from build123d import *

# Parameters (mm, degrees)
SKETCH1_W           = 45
SKETCH1_H           = 6
BOSS_EXTRUDE1_DEPTH = 32
SKETCH2_W           = 23.1
SKETCH2_H           = 17.6
CUT_EXTRUDE1_DEPTH  = 56.542776308
SKETCH3_W           = 45
SKETCH3_H           = 20
BOSS_EXTRUDE2_DEPTH = 6
SKETCH4_W           = 20
SKETCH4_H           = 6
BOSS_EXTRUDE3_DEPTH = 30
SKETCH5_R           = 1.4
CUT_EXTRUDE2_DEPTH  = 87.423376467
BOSS_EXTRUDE4_DEPTH = 7
SKETCH7_W           = 32
SKETCH7_H           = 2.5
CUT_EXTRUDE3_DEPTH  = 17.6
SKETCH8_R           = 1.35
CUT_EXTRUDE4_DEPTH  = 86.895285086
CHAMFER1_SIZE       = 1
FILLET1_R           = 1


with BuildPart() as part:
    # Sketch1 → Boss-Extrude1 (new body)
    with BuildSketch(Plane(origin=(0, 0, 0), x_dir=(1, 0, 0), z_dir=(0, 1, 0))):
        with Locations((22.5, 3)):
            Rectangle(SKETCH1_W, SKETCH1_H)
    extrude(amount=BOSS_EXTRUDE1_DEPTH)

    # Sketch2 → Cut-Extrude1 (cut, through all)
    with BuildSketch(Plane.XY):
        with Locations((22.5, 23.2)):
            Rectangle(SKETCH2_W, SKETCH2_H)
    extrude(amount=-CUT_EXTRUDE1_DEPTH, mode=Mode.SUBTRACT)

    # Sketch3 → Boss-Extrude2 (add)
    with BuildSketch(Plane.XZ):
        with Locations((22.5, -10)):
            Rectangle(SKETCH3_W, SKETCH3_H)
    extrude(amount=BOSS_EXTRUDE2_DEPTH)

    # Sketch4 → Boss-Extrude3 (add)
    with BuildSketch(Plane(origin=(45, 0, 0), x_dir=(0, 0, -1), z_dir=(1, 0, 0))):
        with Locations((10, -3)):
            Rectangle(SKETCH4_W, SKETCH4_H)
    extrude(amount=BOSS_EXTRUDE3_DEPTH)

    # Sketch5 → Cut-Extrude2 (cut, through all)
    with BuildSketch(Plane.XZ.offset(6)):
        with Locations(Location((37.288839919, -16.75, 0), (0, 0, 270))):
            Circle(SKETCH5_R)
        with Locations(Location((47.288839919, -16.75, 0), (0, 0, 270))):
            Circle(SKETCH5_R)
        with Locations(Location((47.288839919, -6.75, 0), (0, 0, 270))):
            Circle(SKETCH5_R)
        with Locations(Location((59.538839919, -16.75, 0), (0, 0, 270))):
            Circle(SKETCH5_R)
        with Locations(Location((71.788839919, -16.75, 0), (0, 0, 270))):
            Circle(SKETCH5_R)
        with Locations(Location((71.788839919, -6.75, 0), (0, 0, 270))):
            Circle(SKETCH5_R)
        with Locations(Location((59.538839919, -6.75, 0), (0, 0, 270))):
            Circle(SKETCH5_R)
    extrude(amount=-CUT_EXTRUDE2_DEPTH, mode=Mode.SUBTRACT)

    # Sketch6 → Boss-Extrude4 (add)
    with BuildSketch(Plane.XY):
        Polygon((0, 32), (0, -6), (45, -6), (45, 0), (45, 32), (34.05, 32), (34.05, 14.4), (10.95, 14.4), (10.95, 32), align=None)
    extrude(amount=BOSS_EXTRUDE4_DEPTH)

    # Sketch7 → Cut-Extrude3 (cut)
    with BuildSketch(Plane(origin=(0, 32, 0), x_dir=(1, 0, 0), z_dir=(0, 1, 0))):
        with Locations((22.5, -1.25)):
            Rectangle(SKETCH7_W, SKETCH7_H)
    extrude(amount=-CUT_EXTRUDE3_DEPTH, mode=Mode.SUBTRACT)

    # Sketch8 → Cut-Extrude4 (cut, through all)
    with BuildSketch(Plane.XY.offset(7)):
        with Locations((8.45, 28)):
            Circle(SKETCH8_R)
        with Locations((36.55, 28)):
            Circle(SKETCH8_R)
    extrude(amount=-CUT_EXTRUDE4_DEPTH, mode=Mode.SUBTRACT)

    # Chamfer1
    chamfer1_edges = [part.edges().sort_by_distance(p)[0] for p in [
        (22.5, -6, 7),
        (0, -6, -6.5),
        (37.5, -6, -20),
        (60, -6, 0),
        (75, -6, -10),
        (45, -6, 3.5),
    ]]
    chamfer(chamfer1_edges, length=CHAMFER1_SIZE)

    # Fillet1
    # the kernel refuses this fillet: 1 mm, written as the material it adds along each edge
    with BuildSketch(Plane(origin=(45, 0, -6), x_dir=(0, 1, 0), z_dir=(0, 0, 1))) as fillet1_piece_1:
        with BuildLine():
            CenterArc((FILLET1_R, -FILLET1_R), FILLET1_R, 90, 90)
            Line((0, -FILLET1_R), (0, 0))
            Line((0, 0), (FILLET1_R, 0))
        make_face()
    extrude(amount=6)
    with BuildSketch(Plane(origin=(45, 0, -6), x_dir=(0, 0, -1), z_dir=(-1, 0, 0))) as fillet1_piece_2:
        with BuildLine():
            CenterArc((FILLET1_R, -FILLET1_R), FILLET1_R, 90, 90)
            Line((0, -FILLET1_R), (0, 0))
            Line((0, 0), (FILLET1_R, 0))
        make_face()
    extrude(amount=45)
    with BuildSketch(Plane(origin=(45, -7.5, 0), x_dir=(1, 0, 0), z_dir=(0, 1, 0))) as fillet1_piece_3_section:
        with BuildLine():
            CenterArc((FILLET1_R, -FILLET1_R), FILLET1_R, 90, 90)
            Line((0, -FILLET1_R), (0, 0))
            Line((0, 0), (FILLET1_R, 0))
        make_face()
    fillet1_piece_3 = extrude(amount=7.5, mode=Mode.PRIVATE)
    fillet1_piece_3 = split(fillet1_piece_3, bisect_by=Plane(origin=(45.042981958, -4.592558865, 0.407441135), z_dir=(0, -0.7071067811865476, 0.7071067811865476)), keep=Keep.TOP, mode=Mode.PRIVATE)
    fillet1_piece_3 = split(fillet1_piece_3, bisect_by=Plane(origin=(45.16446835, -4.83553165, 0.528927527), z_dir=(-0.7071067811865476, 0.7071067811865476, 0)), keep=Keep.TOP, mode=Mode.PRIVATE)
    add(fillet1_piece_3)
    with BuildSketch(Plane(origin=(45, -7.5, 0), x_dir=(1, 0, 0), z_dir=(0, 1, 0))) as fillet1_piece_4_section:
        with BuildLine():
            CenterArc((FILLET1_R, -FILLET1_R), FILLET1_R, 90, 90)
            Line((0, -FILLET1_R), (0, 0))
            Line((0, 0), (FILLET1_R, 0))
        make_face()
    fillet1_piece_4 = extrude(amount=7.5, mode=Mode.PRIVATE)
    fillet1_piece_4 = split(fillet1_piece_4, bisect_by=Plane(origin=(45.528927527, -4.83553165, 0.16446835), z_dir=(0, 0.7071067811865476, -0.7071067811865476)), keep=Keep.TOP, mode=Mode.PRIVATE)
    fillet1_piece_4 = split(fillet1_piece_4, bisect_by=Plane(origin=(45.407441135, -4.592558865, 0.042981958), z_dir=(0.7071067811865476, -0.7071067811865476, 0)), keep=Keep.TOP, mode=Mode.PRIVATE)
    add(fillet1_piece_4)
    with BuildSketch(Plane(origin=(45, -7.5, 0), x_dir=(1, 0, 0), z_dir=(0, 1, 0))) as fillet1_piece_5_section:
        with BuildLine():
            CenterArc((FILLET1_R, -FILLET1_R), FILLET1_R, 90, 90)
            Line((0, -FILLET1_R), (0, 0))
            Line((0, 0), (FILLET1_R, 0))
        make_face()
    fillet1_piece_5 = extrude(amount=7.5, mode=Mode.PRIVATE)
    fillet1_piece_5 = split(fillet1_piece_5, bisect_by=Plane(origin=(45.222376568, -3.546419499, 1.453580501), z_dir=(0, 0.7071067811865476, -0.7071067811865476)), keep=Keep.TOP, mode=Mode.PRIVATE)
    fillet1_piece_5 = split(fillet1_piece_5, bisect_by=Plane(origin=(46.453580501, -3.546419499, 0.222376568), z_dir=(-0.7071067811865476, 0.7071067811865476, 0)), keep=Keep.TOP, mode=Mode.PRIVATE)
    add(fillet1_piece_5)
    with BuildSketch(Plane(origin=(45, 0, -8.5), x_dir=(0, 1, 0), z_dir=(0, 0, 1))) as fillet1_piece_6a_section:
        with BuildLine():
            CenterArc((FILLET1_R, -FILLET1_R), FILLET1_R, 90, 90)
            Line((0, -FILLET1_R), (0, 0))
            Line((0, 0), (FILLET1_R, 0))
        make_face()
    fillet1_piece_6a = extrude(amount=8.5, mode=Mode.PRIVATE)
    fillet1_piece_6a = split(fillet1_piece_6a, bisect_by=Plane(origin=(45.224393795, 0.227043758, -6), z_dir=(0, 0, -1)), keep=Keep.TOP, mode=Mode.PRIVATE)
    fillet1_piece_6a = fillet1_piece_6a - Plane(origin=(47.288839919, 0.227043758, -6.75), x_dir=(0, 0, -1), z_dir=(0, -1, 0)) * Cylinder(1.4, 21, mode=Mode.PRIVATE)
    with BuildSketch(Plane(origin=(47.5, 0, -6), x_dir=(0, 0, -1), z_dir=(-1, 0, 0))) as fillet1_piece_6b_section:
        with BuildLine():
            CenterArc((FILLET1_R, -FILLET1_R), FILLET1_R, 90, 90)
            Line((0, -FILLET1_R), (0, 0))
            Line((0, 0), (FILLET1_R, 0))
        make_face()
    fillet1_piece_6b = extrude(amount=47.5, mode=Mode.PRIVATE)
    fillet1_piece_6b = split(fillet1_piece_6b, bisect_by=Plane(origin=(45, 0.236066937, -6.212082633), z_dir=(1, 0, 0)), keep=Keep.TOP, mode=Mode.PRIVATE)
    fillet1_piece_6b = fillet1_piece_6b - Plane(origin=(47.288839919, 0.236066937, -6.75), x_dir=(0, 0, -1), z_dir=(0, -1, 0)) * Cylinder(1.4, 99, mode=Mode.PRIVATE)
    fillet1_piece_6 = fillet1_piece_6a & fillet1_piece_6b
    add(fillet1_piece_6)
    with BuildSketch(Plane(origin=(45, -7.5, 0), x_dir=(1, 0, 0), z_dir=(0, 1, 0))) as fillet1_piece_7a_section:
        with BuildLine():
            CenterArc((FILLET1_R, -FILLET1_R), FILLET1_R, 90, 90)
            Line((0, -FILLET1_R), (0, 0))
            Line((0, 0), (FILLET1_R, 0))
        make_face()
    fillet1_piece_7a = extrude(amount=10, mode=Mode.PRIVATE)
    fillet1_piece_7a = split(fillet1_piece_7a, bisect_by=Plane(origin=(45.226395114, 0, 0.226395114), z_dir=(0, 1, 0)), keep=Keep.TOP, mode=Mode.PRIVATE)
    with BuildSketch(Plane(origin=(45, 0, -6), x_dir=(0, 1, 0), z_dir=(0, 0, 1))) as fillet1_piece_7b_section:
        with BuildLine():
            CenterArc((FILLET1_R, -FILLET1_R), FILLET1_R, 90, 90)
            Line((0, -FILLET1_R), (0, 0))
            Line((0, 0), (FILLET1_R, 0))
        make_face()
    fillet1_piece_7b = extrude(amount=8.5, mode=Mode.PRIVATE)
    fillet1_piece_7b = split(fillet1_piece_7b, bisect_by=Plane(origin=(45.226395114, 0.226395114, 0), z_dir=(0, 0, 1)), keep=Keep.TOP, mode=Mode.PRIVATE)
    fillet1_piece_7 = fillet1_piece_7a & fillet1_piece_7b
    add(fillet1_piece_7)


solid = part.part
Work out the finished part from the listing and answer in its coordinate system (mm). A direction names the side the tool comes from. Round coordinates to 2 decimals unless told otherwise and drop trailing zeros. Write each loop counter-clockwise with the first axis right and the second up, starting at its lowest first coordinate (ties: lowest second). Pieces come first, ordered by that corner, then holes. Notation, with made-up numbers: (30.25, 38.25) -> (74.25, 38.25) arc R13 ccw to (74.25, 57.25) -> close; hole circle Ø5 at (44.25, -37). An arc over 180 degrees is marked (long way). Answer as CSV lines item,"result". Start each with the question number.
(1) Each of these flat-tipped pins is pushed along its axis until it touches: pin 1 (16 mm diameter, centred on x = 55.5, z = -14.5, fed in from +Y); pin 2 (12 mm diameter, centred on x = 21.5, z = -6, fed in from +Y); pin 3 (4 mm diameter, centred on x = 46.5, y = 16.5, fed in from -Z); pin 4 (1.3 mm diameter, centred on y = 22, z = 4, fed in from -X). Where does it stop, or does it pass through?
(2) The part is cut by section C-C, the plane x = 8.45. Give the vertices of the cut face in (y, z), then the cut area to 3 significant figures.
(3) The mould has two halves that part along Y. Classify faces 1 (the flat face through (34.05, 23, -3)), 2 (the flat face through (23, 14.4, 0)), 3 (the cylindrical face through (8.16, 26.68, -2.96)), 4 (the cylindrical face through (8.16, 26.68, 4.78)): +Y half, -Y half, draft (parallel to the pull), parting line (faces both ways), or undercut.
(4) The part is cut by section D-D, the plane z = 5. Give the vertices of the cut face in (x, y).
(5) The part is cut by section A-A, the plane z = -16.75. Give the vertices of the cut face in (x, y).
(6) Find the intervals of material crossed by probe 1 along X at (y, z) = (-4.2, -16.75); probe 2 along X at (y, z) = (-1.25, -6.75); probe 3 along Z at (x, y) = (10, 28), in increasing order.
(7) A tool of negligible diameter and unlimited length cuts with its end or side. For faces 5 (the flat face through (9, 23, 0)), 6 (the flat face through (22, 13, -6)), 7 (the flat face through (60, -2, 0)), 8 (the flat face through (10.95, 23, 5)), from which of +Z, -Z, +X, -X, +Y, -Y can it reach the whole face along a straight path? Write none if from no direction.
(8) The part is cut by section B-B, the plane y = 28. Give the number of separate pieces and of enclosed holes in the cut face, then the cut area to 3 significant figures.
Output values:
1,pin 1,"stops at y = 0"
1,pin 2,"stops at y = 14.4"
1,pin 3,"stops at z = -6"
1,pin 4,"stops at x = 0"
2,outline,"(-6, -19) -> (-5, -20) -> (0, -20) -> (0, -7) arc R1 cw to (1, -6) -> (26.65, -6) -> (26.65, 0) -> (14.4, 0) -> (14.4, 2.5) -> (26.65, 2.5) -> (26.65, 7) -> (-5, 7) -> (-6, 6) -> close; (29.35, -6) -> (32, -6) -> (32, 0) -> (29.35, 0) -> close; (29.35, 2.5) -> (32, 2.5) -> (32, 7) -> (29.35, 7) -> close"
2,area,"505 mm²"
3,face 1,"draft"
3,face 2,"+Y half"
3,face 3,"undercut"
3,face 4,"undercut"
4,outline,"(0, -5) -> (1, -6) -> (44, -6) -> (45, -5) -> (45, 32) -> (34.05, 32) -> (34.05, 14.4) -> (10.95, 14.4) -> (10.95, 32) -> (0, 32) -> close; hole circle Ø2.7 at (8.45, 28); hole circle Ø2.7 at (36.55, 28)"
5,outline,"(0, -5) -> (1, -6) -> (35.89, -6) -> (35.89, 0) -> (0, 0) -> close; (38.69, -6) -> (45.89, -6) -> (45.89, 0) -> (38.69, 0) -> close; (48.69, -6) -> (58.14, -6) -> (58.14, 0) -> (48.69, 0) -> close; (60.94, -6) -> (70.39, -6) -> (70.39, 0) -> (60.94, 0) -> close; (73.19, -6) -> (74, -6) -> (75, -5) -> (75, 0) -> (73.19, 0) -> close"
6,probe 1,"x = 0 to 35.89, 38.69 to 45.89, 48.69 to 58.14, 60.94 to 70.39, 73.19 to 75"
6,probe 2,"x = 0 to 45.89, 48.69 to 58.14, 60.94 to 70.39, 73.19 to 75"
6,probe 3,"z = -6 to 0, 2.5 to 7"
7,face 5,"+Y"
7,face 6,"-Z, +X, -X, +Y"
7,face 7,"+Z, +X, +Y, -Y"
7,face 8,"+Z, -Z, +Y"
8,separate pieces,"6"
8,enclosed holes,"0"
8,area,"206 mm²"
